Input: part model. Units: mm. Frame: model coordinates. A direction names the side the tool comes from. Round coordinates to 2 decimals unless told otherwise and drop trailing zeros. Loops run counter-clockwise (first coordinate to the right, second up) from the corner with the lowest first, then second, coordinate; pieces in that order, holes last. Notation, with made-up numbers: M -30.5,-6 L 24.5,-6 A19 cw 24.5,29 Z; hole C -28,32.5 d6. An arc over 180 degrees is marked long. Return JSON: item names as keys, results as strings. Group by question number.
1) Section B-B (z = -0.75). Output: boundary loops of the cut face in (x, y), plus the area to 3 significant figures.
2) Material intervals for line 1 (X direction, y = 19.5, z = -2.5); line 2 (X direction, y = 1.5, z = -0.75); line 3 (Y direction, x = -2.5, z = 0.25), sorted ascending. Write a range as from..to.
3) Access query for faces 1 (the face through (7.5, -2, 0)), 2 (the face through (-29.547, 20, -3)), 3 (the face through (10, 3, -3)), 4 (the face through (-22.882, 2.594, -0.021)). Directions: +Z, -Z, +X, -X, +Y, -Y. A direction counts if a zero-diameter tool reaches every point of the face in a straight line with its end or side. Return the directions, or none.
4) Mould query, pull axis Y, two halves, no side actions, for faces 5 (the face through (-25.227, 11.964, -3.226)), 6 (the face through (-29, 22.997, -1)), 7 (the face through (-11, 5, -1.5)), 8 (the face through (-30.5, 13, 0)). Classes: +Y half, -Y half, draft (parallel to the pull), parting line (faces both ways), or undercut.
5) Section A-A (z = -4.25). Output: boundary loops of the cut face in (x, y).
6) Section C-C (y = 16.75). Output: boundary loops of the cut face in (x, z), plus the area to 3 significant figures.
7) Section D-D (x = -18.5). Output: boundary loops of the cut face in (y, z).
8) Contact query for flat-ended pins moving along their axis: P1, Ø1.8, axis at x = 8.5, z = -3, coming from the -Y side; P2, Ø13.5, axis at x = -5, y = 15.5, coming from the -Z side; P3, Ø3.5, axis at y = 4, z = -2.5, coming from the -X side; P4, Ø1.8, axis at y = 21, z = -3, coming from the -X side. Output: stop coordinate, or through.
from build123d import *

# Parameters (mm, degrees)
SKETCH1_W           = 35
SKETCH1_H           = 3
BOSS_EXTRUDE1_DEPTH = 6
BOSS_EXTRUDE2_DEPTH = 3
SKETCH4_W           = 15
SKETCH4_H           = 3
BOSS_EXTRUDE3_DEPTH = 3.5
SKETCH5_W           = 10
SKETCH5_H           = 3
BOSS_EXTRUDE4_DEPTH = 4
SKETCH6_W           = 3
SKETCH6_H           = 10
BOSS_EXTRUDE5_DEPTH = 4


with BuildPart() as part:
    # Sketch1 → Boss-Extrude1 (new body)
    with BuildSketch(Plane(origin=(0, 0, 0), x_dir=(1, 0, 0), z_dir=(0, 1, 0))):
        Rectangle(SKETCH1_W, SKETCH1_H)
    extrude(amount=BOSS_EXTRUDE1_DEPTH)

    # Sketch3 → Boss-Extrude2 (add)
    with BuildSketch(Plane(origin=(0, 0, -1.5), x_dir=(-1, 0, 0), z_dir=(0, 0, -1))):
        Polygon((17.5, 0), (32.547232304, 15.047232304), (32.547232304, 22.997232304), (26.547232304, 22.997232304), (26.547232304, 17.527232304), (15.02, 6), (17.5, 6), align=None)
    extrude(amount=-BOSS_EXTRUDE2_DEPTH)

    # Sketch4 → Boss-Extrude3 (add)
    with BuildSketch(Plane(origin=(0, 0, -1.5), x_dir=(-1, 0, 0), z_dir=(0, 0, -1))):
        with Locations((-10, 4.5)):
            Rectangle(SKETCH4_W, SKETCH4_H)
        Polygon((20.783616152, 11.763616152), (26.547232304, 17.527232304), (26.547232304, 22.997232304), (29.547232304, 22.997232304), (29.547232304, 16.284591617), (20.783616152, 7.520975465), align=None)
    extrude(amount=BOSS_EXTRUDE3_DEPTH)

    # Sketch5 → Boss-Extrude4 (add)
    with BuildSketch(Plane.XZ):
        with Locations((12.5, 0)):
            Rectangle(SKETCH5_W, SKETCH5_H)
    extrude(amount=BOSS_EXTRUDE4_DEPTH)

    # Sketch6 → Boss-Extrude5 (add)
    with BuildSketch(Plane(origin=(-8.75, -8.75, 0), x_dir=(0, 0, 1), z_dir=(-0.707106781, -0.707106781, 0))):
        with Locations((0, 23.014368671)):
            Rectangle(SKETCH6_W, SKETCH6_H)
    extrude(amount=BOSS_EXTRUDE5_DEPTH)


solid = part.part
Returned:
{
 "1": {"outline": "M -32.55,15.05 L -28.56,11.06 L -31.39,8.23 L -24.32,1.16 L -21.49,3.99 L -17.5,0 L 7.5,0 L 7.5,-4 L 17.5,-4 L 17.5,6 L -15.02,6 L -26.55,17.53 L -26.55,23 L -32.55,23 Z", "area": "435 mm^2"},
 "2": {"line 1": "x = -29.55..-26.55", "line 2": "x = -24.66..-23.98, -19..17.5", "line 3": "y = 0..6"},
 "3": {"face 1": "+Z, -Z, -X, -Y", "face 2": "-Z, -X, +Y, -Y", "face 3": "-Z, +X, -X, -Y", "face 4": "+Z, -Z, -Y"},
 "4": {"face 5": "-Y half", "face 6": "+Y half", "face 7": "draft", "face 8": "undercut"},
 "5": {"outline": "M -29.55,16.28 L -20.78,7.52 L -20.78,11.76 L -26.55,17.53 L -26.55,23 L -29.55,23 Z; M 2.5,3 L 17.5,3 L 17.5,6 L 2.5,6 Z"},
 "6": {"outline": "M -32.55,-1.5 L -29.55,-1.5 L -29.55,-5 L -25.77,-5 L -25.77,1.5 L -32.55,1.5 Z", "area": "33.6 mm^2"},
 "7": {"outline": "M 1,-1.5 L 9.48,-1.5 L 9.48,1.5 L 1,1.5 Z"},
 "8": {"P1": "stops at y = 3", "P2": "passes through", "P3": "stops at x = -28.59", "P4": "stops at x = -29.55"}
}
